Verification items for the finished model (mm, model axes). Coordinates: 2 decimals unless noted, no trailing zeros. Order: outer loops, then holes, each group sorted by start corner. A loop starts at its lowest first (then second) coordinate and runs counter-clockwise, first axis right, second up. Notation, with made-up numbers: M 64,37 L 91,37 A21 ccw 91,76 Z; hole C -7,-19 d5. An arc over 180 degrees is marked long. Answer as a JSON object with one key per item and string values. Group by question number.
(1) Cross-section at C-C (z = 7). Enter the section's corners in (x, y), plus the area to 3 significant figures.
(2) Gauge pin test, flat ends, axial feed: pin 1 Ø1 at (y, z) = (-21, 11) entering from -X; pin 2 Ø4 at (x, y) = (33.32, 25.57) entering from +Z; pin 3 Ø1 at (x, z) = (-10.5, 12) entering from +Y. Record the tip position at first contact, or that the pin passes through.
(3) Material ranges on line 1 (Y direction, x = 0, z = 0.8); line 2 (Y direction, x = -42.5, z = 1); line 3 (Z direction, x = -24.5, y = 40.5), recorded low to high.
(4) Cross-section at A-A (y = 0). Enter the section's corners in (x, z).
(5) Mould release check, pull along X, two halves, no side actions. Record for faces 1 (the face through (47.69, 15.02, 10.85)), 2 (the face through (-15.357, 37.428, 0.986)), 3 (the face through (-1, 1, 0)): released by +X, released by -X, zero draft, split by the parting line, or undercut.
from build123d import *

# Parameters (mm, degrees)
F0_R     = 50
F0_R_2   = 1.55
F1_DEPTH = 2
F2_R     = 50
F2_R_2   = 48
F3_DEPTH = 20


with BuildPart() as f1:
    # F0 (on Top) → F1 (new body)
    with BuildSketch(Plane.XY):
        Circle(F0_R)
        with Locations((-25.56798, -33.32084)):
            Circle(F0_R_2, mode=Mode.SUBTRACT)
        with Locations((-33.32084, -25.56798)):
            Circle(F0_R_2, mode=Mode.SUBTRACT)
        with Locations((-29.698485, -29.698485)):
            Circle(F0_R_2, mode=Mode.SUBTRACT)
        with Locations((-16.072704, -38.80294)):
            Circle(F0_R_2, mode=Mode.SUBTRACT)
        with Locations((-10.8704, -40.568885)):
            Circle(F0_R_2, mode=Mode.SUBTRACT)
        with Locations((-5.4821, -41.640684)):
            Circle(F0_R_2, mode=Mode.SUBTRACT)
        with Locations((-21, -36.373067)):
            Circle(F0_R_2, mode=Mode.SUBTRACT)
        with Locations((-38.80294, -16.072704)):
            Circle(F0_R_2, mode=Mode.SUBTRACT)
        with Locations((-36.373067, -21)):
            Circle(F0_R_2, mode=Mode.SUBTRACT)
        with Locations((-40.568885, -10.8704)):
            Circle(F0_R_2, mode=Mode.SUBTRACT)
        with Locations((-41.640684, -5.4821)):
            Circle(F0_R_2, mode=Mode.SUBTRACT)
        with Locations((0, -42)):
            Circle(F0_R_2, mode=Mode.SUBTRACT)
        with Locations((5.4821, -41.640684)):
            Circle(F0_R_2, mode=Mode.SUBTRACT)
        with Locations((10.8704, -40.568885)):
            Circle(F0_R_2, mode=Mode.SUBTRACT)
        with Locations((16.072704, -38.80294)):
            Circle(F0_R_2, mode=Mode.SUBTRACT)
        with Locations((21, -36.373067)):
            Circle(F0_R_2, mode=Mode.SUBTRACT)
        with Locations((25.56798, -33.32084)):
            Circle(F0_R_2, mode=Mode.SUBTRACT)
        with Locations((29.698485, -29.698485)):
            Circle(F0_R_2, mode=Mode.SUBTRACT)
        with Locations((33.32084, -25.56798)):
            Circle(F0_R_2, mode=Mode.SUBTRACT)
        with Locations((36.373067, -21)):
            Circle(F0_R_2, mode=Mode.SUBTRACT)
        with Locations((38.80294, -16.072704)):
            Circle(F0_R_2, mode=Mode.SUBTRACT)
        with Locations((40.568885, -10.8704)):
            Circle(F0_R_2, mode=Mode.SUBTRACT)
        with Locations((41.640684, -5.4821)):
            Circle(F0_R_2, mode=Mode.SUBTRACT)
        with Locations((-42, 0)):
            Circle(F0_R_2, mode=Mode.SUBTRACT)
        with Locations((-41.640684, 5.4821)):
            Circle(F0_R_2, mode=Mode.SUBTRACT)
        with Locations((-40.568885, 10.8704)):
            Circle(F0_R_2, mode=Mode.SUBTRACT)
        with Locations((-38.80294, 16.072704)):
            Circle(F0_R_2, mode=Mode.SUBTRACT)
        with Locations((-36.373067, 21)):
            Circle(F0_R_2, mode=Mode.SUBTRACT)
        with Locations((-33.32084, 25.56798)):
            Circle(F0_R_2, mode=Mode.SUBTRACT)
        with Locations((-29.698485, 29.698485)):
            Circle(F0_R_2, mode=Mode.SUBTRACT)
        with Locations((-25.56798, 33.32084)):
            Circle(F0_R_2, mode=Mode.SUBTRACT)
        with Locations((-21, 36.373067)):
            Circle(F0_R_2, mode=Mode.SUBTRACT)
        with Locations((-16.072704, 38.80294)):
            Circle(F0_R_2, mode=Mode.SUBTRACT)
        with Locations((-10.8704, 40.568885)):
            Circle(F0_R_2, mode=Mode.SUBTRACT)
        with Locations((-5.4821, 41.640684)):
            Circle(F0_R_2, mode=Mode.SUBTRACT)
        with Locations((42, 0)):
            Circle(F0_R_2, mode=Mode.SUBTRACT)
        with Locations((41.640684, 5.4821)):
            Circle(F0_R_2, mode=Mode.SUBTRACT)
        with Locations((40.568885, 10.8704)):
            Circle(F0_R_2, mode=Mode.SUBTRACT)
        with Locations((36.373067, 21)):
            Circle(F0_R_2, mode=Mode.SUBTRACT)
        with Locations((38.80294, 16.072704)):
            Circle(F0_R_2, mode=Mode.SUBTRACT)
        with Locations((21, 36.373067)):
            Circle(F0_R_2, mode=Mode.SUBTRACT)
        with Locations((0, 42)):
            Circle(F0_R_2, mode=Mode.SUBTRACT)
        with Locations((5.4821, 41.640684)):
            Circle(F0_R_2, mode=Mode.SUBTRACT)
        with Locations((10.8704, 40.568885)):
            Circle(F0_R_2, mode=Mode.SUBTRACT)
        with Locations((16.072704, 38.80294)):
            Circle(F0_R_2, mode=Mode.SUBTRACT)
        with Locations((29.698485, 29.698485)):
            Circle(F0_R_2, mode=Mode.SUBTRACT)
        with Locations((33.32084, 25.56798)):
            Circle(F0_R_2, mode=Mode.SUBTRACT)
        with Locations((25.56798, 33.32084)):
            Circle(F0_R_2, mode=Mode.SUBTRACT)
    extrude(amount=F1_DEPTH)

    # F2 (on face) → F3 (join)
    with BuildSketch(Plane.XY.offset(2)):
        Circle(F2_R)
        Circle(F2_R_2, mode=Mode.SUBTRACT)
    extrude(amount=F3_DEPTH)


solid = f1.part
Taken from the geometry:
{
 "1": {"outline": "C 0,0 d100; hole C 0,0 d96", "area": "616 mm²"},
 "2": {"pin 1": "stops at x = -45.6", "pin 2": "stops at z = 2", "pin 3": "stops at y = 48.99"},
 "3": {"line 1": "y = -50 to -43.55, -40.45 to 40.45, 43.55 to 50", "line 2": "y = -26.34 to -6.77, -4.19 to -1.47, 1.47 to 4.19, 6.77 to 26.34", "line 3": "z = 0 to 2"},
 "4": {"outline": "M -50,0 L -43.55,0 L -43.55,2 L -48,2 L -48,22 L -50,22 Z; M -40.45,0 L 40.45,0 L 40.45,2 L -40.45,2 Z; M 43.55,0 L 50,0 L 50,22 L 48,22 L 48,2 L 43.55,2 Z"},
 "5": {"face 1": "split by the parting line", "face 2": "undercut", "face 3": "zero draft"}
}
